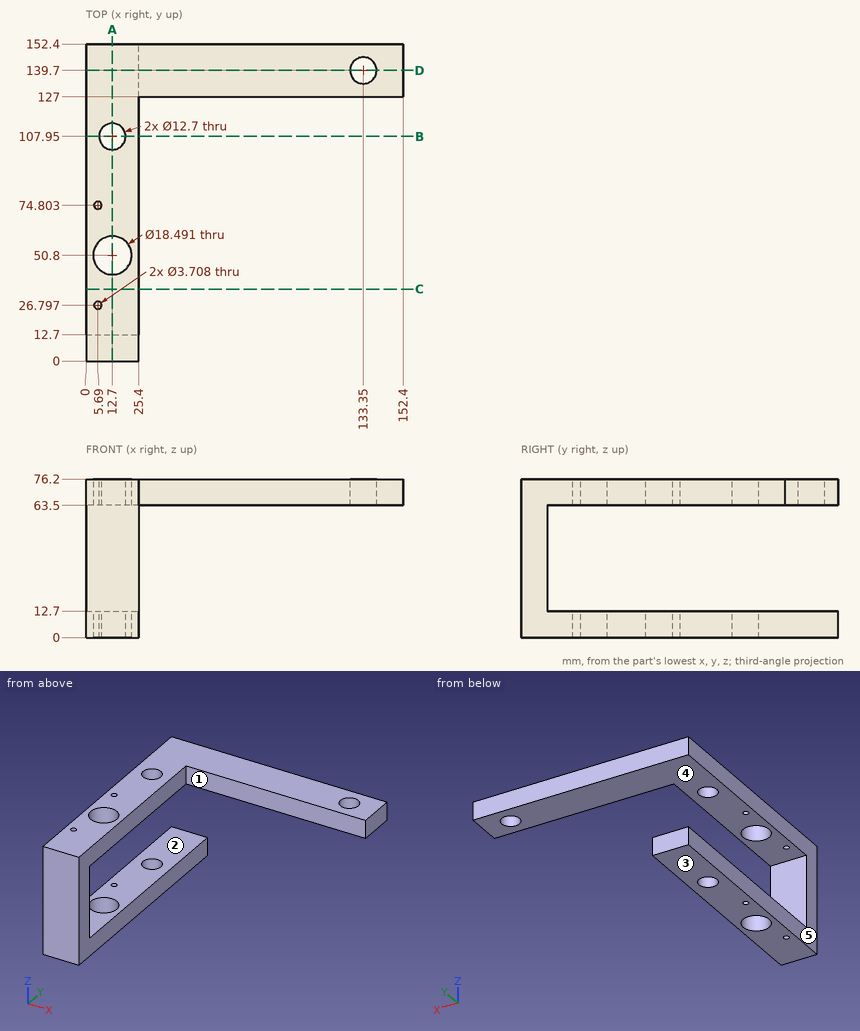
Geometry check sheet. Reference: drawing and pictorial views, mm from the part's lowest x, y, z. A direction names the side the tool comes from. Give positions to 0.01 mm unless a question says otherwise; leave off trailing zeros. Order: outer loops, then holes, each group sorted by start corner. A loop starts at its lowest first (then second) coordinate and runs counter-clockwise, first axis right, second up. Notation, with made-up numbers: M -36.75,16.5 L 20.25,16.5 A29 cw 20.25,45.5 Z; hole C -3.5,21.25 d6. An arc over 180 degrees is marked long. Answer in a Markdown table with one row per item.
1) Cross-section at C-C, the plane y = 34.5. Enter the section's corners in (x, z), plus the area to 3 significant figures.
Filled sheet:
| item | result |
|---|---|
| outline | M 0,0 L 25.4,0 L 25.4,12.7 L 0,12.7 Z; M 0,63.5 L 25.4,63.5 L 25.4,76.2 L 0,76.2 Z |
| area | 645 mm2 |
2) Access from +Z, -Z, +X, -X, +Y, -Y to the whole of each face (thin tool, end or side, straight path). Record for the marked faces 4 and 5.
Filled sheet:
| item | result |
|---|---|
| face 4 | +X, -X, +Y |
| face 5 | +Z, -Z, -X, +Y, -Y |
3) Cross-section at D-D, the plane y = 139.7. Enter the section's corners in (x, z), plus the area to 3 significant figures.
Filled sheet:
| item | result |
|---|---|
| outline | M 0,0 L 25.4,0 L 25.4,12.7 L 0,12.7 Z; M 0,63.5 L 127,63.5 L 127,76.2 L 0,76.2 Z; M 139.7,63.5 L 152.4,63.5 L 152.4,76.2 L 139.7,76.2 Z |
| area | 2,100 mm2 |
4) Release check for a two-part mould opening along Z. For the marked faces 1, 2 and 3 record: +Z half, -Z half, draft (parallel to the pull), parting line (faces both ways), or undercut.
Filled sheet:
| item | result |
|---|---|
| face 1 | draft |
| face 2 | undercut |
| face 3 | -Z half |
5) Gauge pin test, flat ends, axial feed: P1, Ø3, axis at x = 76.5, y = 128, coming from the -Z side; P2, Ø6, axis at x = 28, z = 53, coming from the +Y side; P3, Ø4, axis at x = 73.5, z = 68.5, coming from the -Y side. Record the tip position at first contact, or that the pin passes through.
Filled sheet:
| item | result |
|---|---|
| P1 | stops at z = 63.5 |
| P2 | stops at y = 12.7 |
| P3 | stops at y = 127 |
6) Cross-section at B-B, the plane y = 107.95. Enter the section's corners in (x, z).
Filled sheet:
| item | result |
|---|---|
| outline | M 0,0 L 6.35,0 L 6.35,12.7 L 0,12.7 Z; M 0,63.5 L 6.35,63.5 L 6.35,76.2 L 0,76.2 Z; M 19.05,0 L 25.4,0 L 25.4,12.7 L 19.05,12.7 Z; M 19.05,63.5 L 25.4,63.5 L 25.4,76.2 L 19.05,76.2 Z |
7) Thickness scan on L1, parallel to Y at x = 12.7, z = 69.75 (1 decimal); L2, parallel to X at y = 50.8, z = 6.25 (1 decimal); L3, parallel to Z at x = 139.5, y = 143. Record the ranges inside material, lowest first. Write a range as [from, to].
Filled sheet:
| item | result |
|---|---|
| L1 | y = [0, 41.6], [60, 101.6], [114.3, 152.4] |
| L2 | x = [0, 3.5], [21.9, 25.4] |
| L3 | z = [63.5, 76.2] |
8) Cross-section at A-A, the plane x = 12.7. Enter the section's corners in (y, z) (1 decimal), plus the area to 3 significant figures.
Filled sheet:
| item | result |
|---|---|
| outline | M 0,0 L 41.6,0 L 41.6,12.7 L 12.7,12.7 L 12.7,63.5 L 41.6,63.5 L 41.6,76.2 L 0,76.2 Z; M 60,0 L 101.6,0 L 101.6,12.7 L 60,12.7 Z; M 60,63.5 L 101.6,63.5 L 101.6,76.2 L 60,76.2 Z; M 114.3,0 L 152.4,0 L 152.4,12.7 L 114.3,12.7 Z; M 114.3,63.5 L 152.4,63.5 L 152.4,76.2 L 114.3,76.2 Z |
| area | 3,720 mm2 |
